Model file for the job. Use its own axes, mm. Face numbers are marked on the shaded views. A direction names the side the tool comes from. Coordinates: 2 decimals unless noted, no trailing zeros. Loops run counter-clockwise (first coordinate to the right, second up) from the corner with the lowest first, then second, coordinate; pieces in that order, holes last.
from build123d import *

# Parameters (mm, degrees)
BOSS_EXTRUDE1_DEPTH     = 15.5
SKETCH10_W              = 4
SKETCH10_H              = 30
CUT_EXTRUDE1_DEPTH      = 3
MIRROR5_COPY_1_SKETCH_W = 4
MIRROR5_COPY_1_SKETCH_H = 30
MIRROR5_COPY_1_DEPTH    = 3
SKETCH14_W              = 2.751713212
SKETCH14_H              = 4
BOSS_EXTRUDE2_DEPTH     = 4
SKETCH15_W              = 4.497862048
SKETCH15_H              = 7
BOSS_EXTRUDE3_DEPTH     = 1
MIRROR7_COPY_1_SKETCH_W = 2.751713212
MIRROR7_COPY_1_SKETCH_H = 4
MIRROR7_COPY_1_DEPTH    = 4
MIRROR7_COPY_2_SKETCH_W = 4.497862048
MIRROR7_COPY_2_SKETCH_H = 7
MIRROR7_COPY_2_DEPTH    = 1
CHAMFER9_SIZE           = 5
CHAMFER10_SIZE          = 1
CHAMFER15_SIZE          = 5
CHAMFER16_SIZE          = 1
CHAMFER17_SIZE          = 1
CHAMFER18_SIZE          = 5
CHAMFER19_SIZE          = 1


with BuildPart() as part:
    # Sketch1 → Boss-Extrude1 (new body)
    with BuildSketch(Plane(origin=(0, 0, 0), x_dir=(1, 0, 0), z_dir=(0, 1, 0))):
        Polygon((-106.77339112, 72.768445428), (-99.77339112, 72.768445428), (-99.77339112, 56.768445428), (-86.77339112, 56.768445428), (-86.77339112, 72.768445428), (-76.77339112, 72.768445428), (-76.77339112, 56.768445428), (-63.77339112, 56.768445428), (-63.77339112, 72.768445428), (-53.77339112, 72.768445428), (-53.77339112, 56.768445428), (-40.77339112, 56.768445428), (-40.77339112, 72.768445428), (-30.77339112, 72.768445428), (-30.77339112, 56.768445428), (-17.77339112, 56.768445428), (-17.77339112, 72.768445428), (-10.77339112, 72.768445428), (-10.77339112, 7.054306764), (-34.835725148, -23.581828326), (-30.98324076, -26.60765929), (-38.753655744, -36.500942414), (-30.205167067, -43.215124519), (-30.205167067, -57.231554572), (-106.77339112, -57.231554572), align=None)
    extrude(amount=BOSS_EXTRUDE1_DEPTH)

    # Sketch4 → Revolve1 (revolve)
    with BuildSketch(Plane(origin=(-99.77339112, 0, 0), x_dir=(0, 0, -1), z_dir=(1, 0, 0))):
        with BuildLine():
            Line((67.768445428, 8), (71.768445428, 8))
            ThreePointArc((71.768445428, 8), (69.768445428, 10), (67.768445428, 8))
        make_face()
    revolve1 = revolve(axis=Axis((-99.77339112, 8, -67.768445428), (0, 0, -1)))

    # Mirror1: Revolve1 across plane
    add(revolve1.mirror(Plane(origin=(-93.27339112, 0, 0), x_dir=(0, 0, 1), z_dir=(1, 0, 0))))

    # Mirror2: Revolve1 across plane
    add(revolve1.mirror(Plane(origin=(-81.77339112, 0, 0), x_dir=(0, 0, 1), z_dir=(1, 0, 0))))

    # Mirror2 copy 1 sketch → Mirror2 copy 1 (revolve)
    with BuildSketch(Plane(origin=(-76.77339112, 0, 0), x_dir=(0, 0, -1), z_dir=(1, 0, 0))):
        with BuildLine():
            Line((67.768445428, 8), (71.768445428, 8))
            ThreePointArc((71.768445428, 8), (69.768445428, 10), (67.768445428, 8))
        make_face()
    revolve(axis=Axis((-76.77339112, 8, -67.768445428), (0, 0, -1)))

    # Mirror3: Revolve1 across plane
    add(revolve1.mirror(Plane(origin=(-58.77339112, 0, 0), x_dir=(0, 0, 1), z_dir=(1, 0, 0))))

    # Mirror3 copy 1 sketch → Mirror3 copy 1 (revolve)
    with BuildSketch(Plane(origin=(-53.77339112, 0, 0), x_dir=(0, 0, -1), z_dir=(1, 0, 0))):
        with BuildLine():
            Line((67.768445428, 8), (71.768445428, 8))
            ThreePointArc((71.768445428, 8), (69.768445428, 10), (67.768445428, 8))
        make_face()
    revolve(axis=Axis((-53.77339112, 8, -67.768445428), (0, 0, -1)))

    # Mirror3 copy 2 sketch → Mirror3 copy 2 (revolve)
    with BuildSketch(Plane(origin=(-40.77339112, 0, 0), x_dir=(0, 0, -1), z_dir=(-1, 0, 0))):
        with BuildLine():
            Line((67.768445428, -8), (71.768445428, -8))
            ThreePointArc((71.768445428, -8), (69.768445428, -10), (67.768445428, -8))
        make_face()
    revolve(axis=Axis((-40.77339112, 8, -67.768445428), (0, 0, 1)))

    # Mirror3 copy 3 sketch → Mirror3 copy 3 (revolve)
    with BuildSketch(Plane(origin=(-30.77339112, 0, 0), x_dir=(0, 0, -1), z_dir=(1, 0, 0))):
        with BuildLine():
            Line((67.768445428, 8), (71.768445428, 8))
            ThreePointArc((71.768445428, 8), (69.768445428, 10), (67.768445428, 8))
        make_face()
    revolve(axis=Axis((-30.77339112, 8, -67.768445428), (0, 0, -1)))

    # Sketch10 → Cut-Extrude1 (cut)
    with BuildSketch(Plane(origin=(0, -17.5, -17.5), x_dir=(-1, 0, 0), z_dir=(0, -0.707106781, -0.707106781))):
        with Locations((24.27339112, 40.141352719)):
            Rectangle(SKETCH10_W, SKETCH10_H)
    cut_extrude1 = extrude(amount=CUT_EXTRUDE1_DEPTH, mode=Mode.SUBTRACT)

    # Mirror4: Cut-Extrude1 across plane
    add(cut_extrude1.mirror(Plane(origin=(-35.77339112, 0, 0), x_dir=(0, 0, 1), z_dir=(1, 0, 0))), mode=Mode.SUBTRACT)

    # Mirror5: Cut-Extrude1 across plane
    add(cut_extrude1.mirror(Plane(origin=(-58.77339112, 0, 0), x_dir=(0, 0, 1), z_dir=(1, 0, 0))), mode=Mode.SUBTRACT)

    # Mirror5 copy 1 sketch → Mirror5 copy 1 (cut)
    with BuildSketch(Plane(origin=(-46, -17.5, -17.5), x_dir=(-1, 0, 0), z_dir=(0, -0.707106781, -0.707106781))):
        with Locations((24.27339112, 40.141352719)):
            Rectangle(MIRROR5_COPY_1_SKETCH_W, MIRROR5_COPY_1_SKETCH_H)
    extrude(amount=MIRROR5_COPY_1_DEPTH, mode=Mode.SUBTRACT)

    # Sketch14 → Boss-Extrude2 (add)
    with BuildSketch(Plane(origin=(0, 0, 0), x_dir=(-1, 0, 0), z_dir=(0, -1, 0))):
        with Locations((24.227451545, 51.242640687)):
            Rectangle(SKETCH14_W, SKETCH14_H)
    boss_extrude2 = extrude(amount=BOSS_EXTRUDE2_DEPTH)

    # Sketch15 → Boss-Extrude3 (add)
    with BuildSketch(Plane.XZ.offset(4)):
        with Locations((-24.227451545, -51.242640687)):
            Rectangle(SKETCH15_W, SKETCH15_H)
    boss_extrude3 = extrude(amount=BOSS_EXTRUDE3_DEPTH)

    # Mirror6: Boss-Extrude2, Boss-Extrude3 across plane
    add(boss_extrude2.mirror(Plane(origin=(-35.77339112, 0, 0), x_dir=(0, 0, 1), z_dir=(1, 0, 0))))
    add(boss_extrude3.mirror(Plane(origin=(-35.77339112, 0, 0), x_dir=(0, 0, 1), z_dir=(1, 0, 0))))

    # Mirror7: Boss-Extrude2, Boss-Extrude3 across plane
    add(boss_extrude2.mirror(Plane(origin=(-58.77339112, 0, 0), x_dir=(0, 0, 1), z_dir=(1, 0, 0))))
    add(boss_extrude3.mirror(Plane(origin=(-58.77339112, 0, 0), x_dir=(0, 0, 1), z_dir=(1, 0, 0))))

    # Mirror7 copy 1 sketch → Mirror7 copy 1 (add)
    with BuildSketch(Plane(origin=(-46, 0, 0), x_dir=(-1, 0, 0), z_dir=(0, -1, 0))):
        with Locations((24.227451545, 51.242640687)):
            Rectangle(MIRROR7_COPY_1_SKETCH_W, MIRROR7_COPY_1_SKETCH_H)
    extrude(amount=MIRROR7_COPY_1_DEPTH)

    # Mirror7 copy 2 sketch → Mirror7 copy 2 (add)
    with BuildSketch(Plane(origin=(-46, -4, 0), x_dir=(1, 0, 0), z_dir=(0, -1, 0))):
        with Locations((-24.227451545, -51.242640687)):
            Rectangle(MIRROR7_COPY_2_SKETCH_W, MIRROR7_COPY_2_SKETCH_H)
    extrude(amount=MIRROR7_COPY_2_DEPTH)

    # Chamfer9
    chamfer9_edges = [part.edges().sort_by_distance(p)[0] for p in [
        (-103.27339112, 15.5, -72.768445428),
    ]]
    chamfer(chamfer9_edges, length=CHAMFER9_SIZE)

    # Chamfer10
    chamfer10_edges = [part.edges().sort_by_distance(p)[0] for p in [
        (-99.77339112, 15.5, -62.268445428),
        (-99.77339112, 13, -70.268445428),
    ]]
    chamfer(chamfer10_edges, length=CHAMFER10_SIZE)

    # Chamfer15
    chamfer15_edges = [part.edges().sort_by_distance(p)[0] for p in [
        (-81.77339112, 15.5, -72.768445428),
    ]]
    chamfer(chamfer15_edges, length=CHAMFER15_SIZE)

    # Chamfer16
    chamfer16_edges = [part.edges().sort_by_distance(p)[0] for p in [
        (-86.77339112, 13, -70.268445428),
        (-86.77339112, 15.5, -62.268445428),
    ]]
    chamfer(chamfer16_edges, length=CHAMFER16_SIZE)

    # Chamfer17
    chamfer17_edges = [part.edges().sort_by_distance(p)[0] for p in [
        (-76.77339112, 15.5, -62.268445428),
        (-76.77339112, 13, -70.268445428),
    ]]
    chamfer(chamfer17_edges, length=CHAMFER17_SIZE)

    # Chamfer18
    chamfer18_edges = [part.edges().sort_by_distance(p)[0] for p in [
        (-14.27339112, 15.5, -72.768445428),
        (-35.77339112, 15.5, -72.768445428),
        (-58.77339112, 15.5, -72.768445428),
    ]]
    chamfer(chamfer18_edges, length=CHAMFER18_SIZE)

    # Chamfer19
    chamfer19_edges = [part.edges().sort_by_distance(p)[0] for p in [
        (-17.77339112, 15.5, -62.268445428),
        (-40.77339112, 15.5, -62.268445428),
        (-30.77339112, 15.5, -62.268445428),
        (-53.77339112, 15.5, -62.268445428),
        (-17.77339112, 13, -70.268445428),
        (-30.77339112, 13, -70.268445428),
        (-40.77339112, 13, -70.268445428),
        (-53.77339112, 13, -70.268445428),
        (-63.77339112, 13, -70.268445428),
        (-63.77339112, 15.5, -62.268445428),
    ]]
    chamfer(chamfer19_edges, length=CHAMFER19_SIZE)


solid = part.part
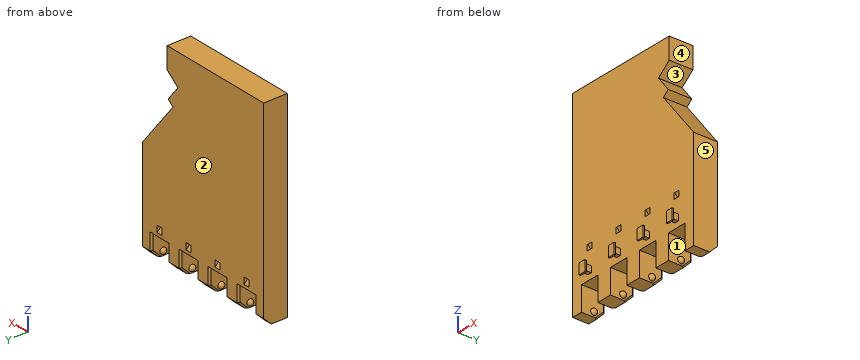
Q1. Slice it at B-B (z = -13.5). List the corners of the cut face in (x, y).
Answers:
outline: (-106.77, 0) - (-10.77, 0) - (-10.77, 15.5) - (-106.77, 15.5) - close
Q2. Slice it at A-A (z = -45). List the corners of the cut face in (x, y).
Answers:
outline: (-106.77, 0) - (-10.77, 0) - (-10.77, 15.5) - (-106.77, 15.5) - close; hole (-95.27, 5.76) - (-91.27, 5.76) - (-91.27, 10) - (-95.27, 10) - close; hole (-72.27, 5.76) - (-68.27, 5.76) - (-68.27, 10) - (-72.27, 10) - close; hole (-49.27, 5.76) - (-45.27, 5.76) - (-45.27, 10) - (-49.27, 10) - close; hole (-26.27, 5.76) - (-22.27, 5.76) - (-22.27, 10) - (-26.27, 10) - close
Q3. Slice it at C-C (y = 12.25). Count the separate pieces of the cut face and the enclosed holes in it, and give its area (3 significant figures).
Answers:
separate pieces: 1
enclosed holes: 4
area: 10,400 mm2
Q4. Mould opens along X. For the marked faces 1, 2 and 3 say: +X half, -X half, draft (parallel to the pull), parting line (faces both ways), or undercut.
Answers:
face 1: undercut
face 2: draft
face 3: +X half
Q5. Flat gauge pins, fed straight in: P1, Ø2, axis at x = -93.5, y = -2, coming from the -Z side; P2, Ø12, axis at x = -22.5, z = -0.5, coming from the -Y side; P3, Ø1, axis at x = -68.5, y = 8.5, coming from the -Z side. Where does each tip first touch, or does it go through?
Answers:
P1: stops at z = -53.24
P2: stops at y = 0
P3: stops at z = -56.77
Q6. Which spindle directions (+Z, -Z, +X, -X, +Y, -Y) get a long thin tool onto all of the face, cutting with end or side? Do the marked faces 4 and 5. Say none if no direction does.
Answers:
face 4: +Z, +X, +Y, -Y
face 5: +Z, -Z, +X, +Y, -Y
Q7. Drill centre lines: line 1 (X direction, y = 5.25, z = -61); line 2 (Z direction, x = -30.5, y = 7); line 3 (Z direction, x = -70, y = -2.25). Where is each one in solid material? Low to high.
Answers:
line 1: x = -106.77 to -99.77, -86.77 to -76.77, -63.77 to -53.77, -40.77 to -30.77, -17.77 to -10.77
line 2: z = -71.48 to -68.06, -56.77 to 18.06, 42.98 to 57.23
line 3: z = -53.24 to -49.24
